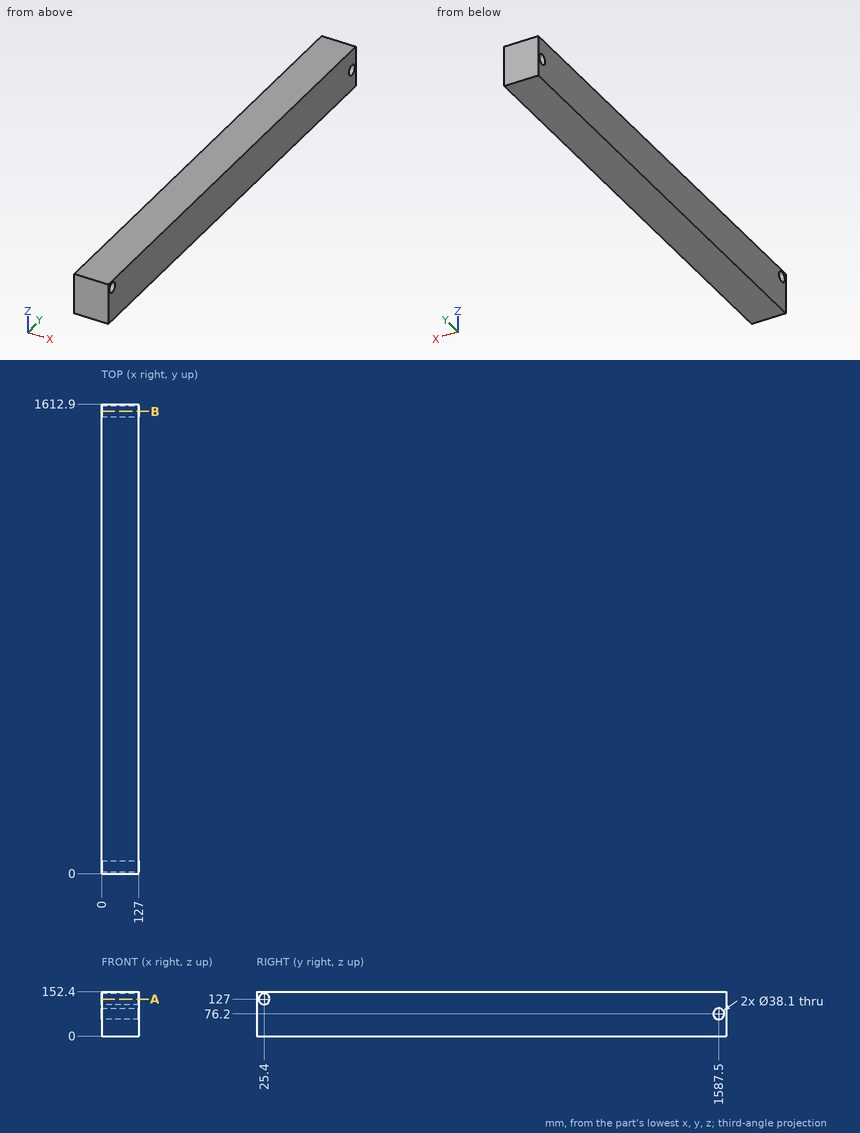
Part print with two shaded views. Sizes in mm from the minimum x, y, z corner. Round coordinates to 2 decimals unless told otherwise and drop trailing zeros. Order: outer loops, then holes, each group sorted by start corner. A loop starts at its lowest first (then second) coordinate and runs counter-clockwise, first axis right, second up.
(1) Band-saw the part on A-A (z = 127). List the corners of the cut face in (x, y).
(2) Band-saw the part on B-B (y = 1587.5). List the corners of the cut face in (x, z), then the cut area to 3 significant figures.
(3) Drill centre lines: line 1 (Y direction, x = 43, z = 76); line 2 (Z direction, x = 87, y = 1587.5); line 3 (Y direction, x = 31, z = 127). Where is each one in solid material? Low to high.
(4) Pin check, flat tip, straight feed: pin 1 (23 mm diameter, centred on y = 25.4, z = 127, fed in from -X). Stop position of the tip, or through.
Verdict:
1. outline: (0, 0) - (127, 0) - (127, 6.35) - (0, 6.35) - close; (0, 44.45) - (127, 44.45) - (127, 1612.9) - (0, 1612.9) - close
2. outline: (0, 0) - (127, 0) - (127, 57.15) - (0, 57.15) - close; (0, 95.25) - (127, 95.25) - (127, 152.4) - (0, 152.4) - close
2. area: 14,500 mm2
3. line 1: y = 0 to 1568.45, 1606.55 to 1612.9
3. line 2: z = 0 to 57.15, 95.25 to 152.4
3. line 3: y = 0 to 6.35, 44.45 to 1612.9
4. pin 1: passes through
